Geometry check sheet. Reference: the model listing, model coordinates, mm. Face numbers are marked on the shaded views. A direction names the side the tool comes from. Coordinates: 2 decimals unless noted, no trailing zeros. Write each loop counter-clockwise with the first axis right and the second up, starting at its lowest first coordinate (ties: lowest second). Pieces come first, ordered by that corner, then holes. Notation, with made-up numbers: (-29.5, -28.75) - (10.5, -28.75) arc R20 ccw to (10.5, -5.75) - close; hole circle Ø6 at (53.5, -39.5). An arc over 180 degrees is marked (long way). Answer as a JSON object with one key per item and string values. Group by question number.
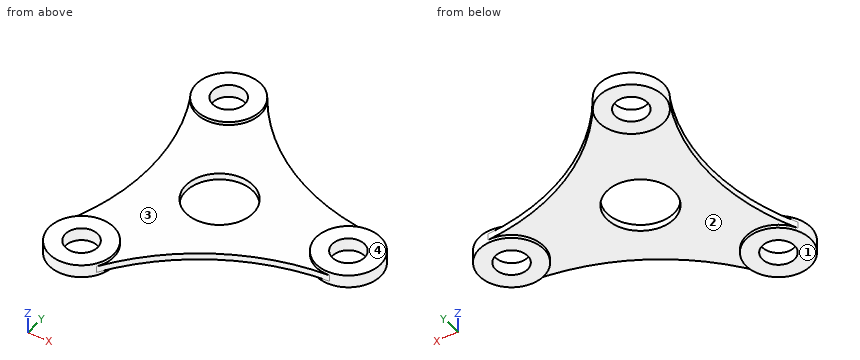
from build123d import *

# Parameters (mm, degrees)
SKETCH1_R             = 50
SKETCH1_R_2           = 25
BOSS_EXTRUDE1_DEPTH   = 10
BOSS_EXTRUDE1_2_DEPTH = 10
BOSS_EXTRUDE1_3_DEPTH = 10
SKETCH1_3_R           = 52
BOSS_EXTRUDE2_DEPTH   = 5


with BuildPart() as part:
    # Sketch1 → Boss-Extrude1 (new, symmetric)
    with BuildSketch(Plane.XY):
        with Locations((-100, 173.205080757)):
            Circle(SKETCH1_R)
        with Locations((-100, 173.205080757)):
            Circle(SKETCH1_R_2, mode=Mode.SUBTRACT)
    extrude(amount=BOSS_EXTRUDE1_DEPTH, both=True)



with BuildPart() as body_2:
    # Sketch1 → Boss-Extrude1 2 (new, symmetric)
    with BuildSketch(Plane.XY):
        with Locations((-100, -173.205080757)):
            Circle(SKETCH1_R)
        with Locations((-100, -173.205080757)):
            Circle(SKETCH1_R_2, mode=Mode.SUBTRACT)
    extrude(amount=BOSS_EXTRUDE1_2_DEPTH, both=True)


with BuildPart() as body_3:
    # Sketch1 → Boss-Extrude1 3 (new, symmetric)
    with BuildSketch(Plane.XY):
        with Locations((200, 0)):
            Circle(SKETCH1_R)
        with Locations((200, 0)):
            Circle(SKETCH1_R_2, mode=Mode.SUBTRACT)
    extrude(amount=BOSS_EXTRUDE1_3_DEPTH, both=True)


with BuildPart() as part_1:
    add(part.part)

    add(body_2.part)  # Boss-Extrude2 merges body 2

    add(body_3.part)  # Boss-Extrude2 merges body 3
    # Sketch1<3> → Boss-Extrude2 (add, symmetric)
    with BuildSketch(Plane.XY):
        with BuildLine():
            ThreePointArc((203.542445822, -49.874352904), (150, 0), (203.542445822, 49.874352904))
            ThreePointArc((203.542445822, 49.874352904), (55.056170912, 95.360085291), (-58.578766299, 201.210105283))
            ThreePointArc((-58.578766299, 201.210105283), (-52.19277416, 187.849846288), (-50, 173.205080757))
            ThreePointArc((-50, 173.205080757), (-88.779126063, 124.480425929), (-144.963679523, 151.335752378))
            ThreePointArc((-144.963679523, 151.335752378), (-110.112341825, 0), (-144.963679523, -151.335752378))
            ThreePointArc((-144.963679523, -151.335752378), (-88.779126063, -124.480425929), (-50, -173.205080757))
            ThreePointArc((-50, -173.205080757), (-52.19277416, -187.849846288), (-58.578766299, -201.210105283))
            ThreePointArc((-58.578766299, -201.210105283), (55.056170912, -95.360085291), (203.542445822, -49.874352904))
        make_face()
        Circle(SKETCH1_3_R, mode=Mode.SUBTRACT)
    extrude(amount=BOSS_EXTRUDE2_DEPTH, both=True)


solid = part_1.part
(1) Draft check along Y on the marked faces 3 and 4. Enter one of: +Y half, -Y half, draft (parallel to the pull), parting line (faces both ways), or undercut.
(2) Section check B-B (y = 0). Record the cut outline in (x, z), and give its area (3 significant figures).
(3) Gauge pin test, flat ends, axial feed: pin 1 (4 mm diameter, centred on x = 16.5, y = 86, fed in from +Z); pin 2 (6 mm diameter, centred on x = 33.5, z = -5.5, fed in from -Y); pin 3 (1 mm diameter, centred on x = -85.5, z = 0, fed in from -Y). Record the tip position at first contact, or that the pin passes through.
(4) Section check A-A (x = -100). Record the cut outline in (y, z), and give its area (3 significant figures).
(5) Section check D-D (x = 0). Record the cut outline in (y, z), and give its area (3 significant figures).
(6) Material ranges on L1, parallel to Y at x = -100, z = 2; L2, parallel to X at y = 174.5, z = -8.5; L3, parallel to Z at x = -65, y = -45, recorded low to high. Write a range as [from, to].
(7) Set-up check for the marked faces 1 and 2: record each of +Z, -Z, +X, -X, +Y, -Y from which the full face is reachable in a straight line by a thin tool's end or side.
(8) Section check C-C (z = 1.5). Record the cut outline in (x, y).
Conclusion:
{
 "1": {"face 3": "undercut", "face 4": "draft"},
 "2": {"outline": "(-110.11, -5) - (-52, -5) - (-52, 5) - (-110.11, 5) - close; (52, -5) - (150, -5) - (150, -10) - (175, -10) - (175, 10) - (150, 10) - (150, 5) - (52, 5) - close; (225, -10) - (250, -10) - (250, 10) - (225, 10) - close", "area": "2,560 mm^2"},
 "3": {"pin 1": "stops at z = 5", "pin 2": "stops at y = -110.92", "pin 3": "stops at y = -221.21"},
 "4": {"outline": "(-223.21, -10) - (-198.21, -10) - (-198.21, 10) - (-223.21, 10) - close; (-148.21, -10) - (-123.21, -10) - (-123.21, -5) - (123.21, -5) - (123.21, -10) - (148.21, -10) - (148.21, 10) - (123.21, 10) - (123.21, 5) - (-123.21, 5) - (-123.21, 10) - (-148.21, 10) - close; (198.21, -10) - (223.21, -10) - (223.21, 10) - (198.21, 10) - close", "area": "4,460 mm^2"},
 "5": {"outline": "(-134.8, -5) - (-52, -5) - (-52, 5) - (-134.8, 5) - close; (52, -5) - (134.8, -5) - (134.8, 5) - (52, 5) - close", "area": "1,660 mm^2"},
 "6": {"L1": "y = [-223.21, -198.21], [-148.21, 148.21], [198.21, 223.21]", "L2": "x = [-149.98, -124.97], [-75.03, -50.02]", "L3": "z = [-5, 5]"},
 "7": {"face 1": "-Z, +X, -X, +Y, -Y", "face 2": "-Z"},
 "8": {"outline": "(-144.96, -151.34) arc R50 ccw to (-58.58, -201.21) arc R346 cw to (203.54, -49.87) arc R50 ccw to (203.54, 49.87) arc R346 cw to (-58.58, 201.21) arc R50 ccw to (-144.96, 151.34) arc R346 cw to start; hole circle Ø50 at (-100, -173.21); hole circle Ø50 at (-100, 173.21); hole circle Ø104 at (0, 0); hole circle Ø50 at (200, 0)"}
}
